Could you check a few things on this model? Use its own coordinates, in mm. Face numbers are marked on the shaded views. A direction names the side the tool comes from. Round coordinates to 2 decimals unless told otherwise and drop trailing zeros. Loops run counter-clockwise (first coordinate to the right, second up) from the corner with the lowest first, then second, coordinate; pieces in that order, holes last. Notation, with made-up numbers: (77, -36) -> (89, -36) arc R18 ccw to (89, -21) -> close; hole circle Ø5 at (64, 45.5). An arc over 180 degrees is marked (long way). One line per item, written item: value.
```python
from build123d import *

# Parameters (mm, degrees)
SKETCH2_R              = 1.5
BOSS_EXTRUDE1_DEPTH    = 8
CHAMFER1_SIZE          = 0.375
CUT_SWEEP1_PITCH       = 0.5
CUT_SWEEP1_HEIGHT      = 8.5
CUT_SWEEP1_RADIUS      = 1.5
CUT_SWEEP1_START_ANGLE = -90
CUT_EXTRUDE1_DEPTH     = 1.62
SKETCH8_R              = 1.154700538
CUT_EXTRUDE2_DEPTH     = 11.0000001
CUT_EXTRUDE2_DRAFT     = -45
SKETCH9_R              = 1.5
BOSS_EXTRUDE2_DEPTH    = 8.38
CHAMFER2_SIZE          = 0.5
CHAMFER2_SIZE2         = 0.866025404


with BuildPart() as part:
    # Sketch2 → Boss-Extrude1 (new body)
    with BuildSketch(Plane(origin=(4, 0, 0), x_dir=(0, 0, -1), z_dir=(1, 0, 0))):
        Circle(SKETCH2_R)
    extrude(amount=-BOSS_EXTRUDE1_DEPTH)

    # Chamfer1
    chamfer1_edges = [part.edges().sort_by_distance(p)[0] for p in [
        (4, 0, 1.5),
    ]]
    chamfer(chamfer1_edges, length=CHAMFER1_SIZE)

    # Cut-Sweep1: sweep along a helix
    with BuildLine() as cut_sweep1_path:
        add(Helix(CUT_SWEEP1_PITCH, CUT_SWEEP1_HEIGHT, CUT_SWEEP1_RADIUS, center=(4, 0, 0), direction=(-1, 0, 0), mode=Mode.PRIVATE).rotate(Axis((4, 0, 0), (-1, 0, 0)), CUT_SWEEP1_START_ANGLE))
    # Sketch5 → Cut-Sweep1 (sweep, cut)
    with BuildSketch(Plane.XY):
        Polygon((3.78125, 1.5), (4.21875, 1.5), (4.03125, 1.175240474), (3.96875, 1.175240474), align=None)
    sweep(path=cut_sweep1_path.line, is_frenet=True, mode=Mode.SUBTRACT)

    # Sketch6 → Revolve1 (revolve)
    with BuildSketch(Plane.XY):
        Polygon((-5.75, 2.75), (-6, 2.5), (-6, 0), (-4, 0), (-4, 2.75), align=None)
    revolve(axis=Axis((-4, 0, 0), (-1, 0, 0)))

    # Sketch4 → Cut-Extrude1 (cut)
    with BuildSketch(Plane(origin=(-6, 0, 0), x_dir=(0, 0, -1), z_dir=(1, 0, 0))):
        Polygon((0, 1.154700538), (-1, 0.577350269), (-1, -0.577350269), (0, -1.154700538), (1, -0.577350269), (1, 0.577350269), align=None)
    extrude(amount=CUT_EXTRUDE1_DEPTH, mode=Mode.SUBTRACT)


with BuildPart() as cut_extrude2_tool:
    # Sketch8 → Cut-Extrude2 (with draft: the straight prism first)
    with BuildSketch(Plane.ZY.offset(6)):
        Circle(SKETCH8_R)
    extrude(amount=-CUT_EXTRUDE2_DEPTH)
    # Cut-Extrude2: the draft: its side faces are tilted about the plane it starts from
    cut_extrude2_sides = [cut_extrude2_tool.faces().sort_by_distance(p)[0] for p in [
        (-0.49999995, 0, -1.154700538),
    ]]
    draft(cut_extrude2_sides, Plane.ZY.offset(6), CUT_EXTRUDE2_DRAFT)


with BuildPart() as part_1:
    add(part.part)

    # Cut-Extrude2: cut by cut_extrude2_tool
    add(cut_extrude2_tool.part, mode=Mode.SUBTRACT)

    # Sketch9 → Boss-Extrude2 (add)
    with BuildSketch(Plane(origin=(4, 0, 0), x_dir=(0, 0, -1), z_dir=(1, 0, 0))):
        Circle(SKETCH9_R)
    extrude(amount=-BOSS_EXTRUDE2_DEPTH)

    # Chamfer2
    chamfer2_edges = [part_1.edges().sort_by_distance(p)[0] for p in [
        (4, 0, 1.5),
    ]]
    chamfer2_side = [part_1.faces().sort_by_distance(p)[0] for p in [
        (0, 0, 1.5),
    ]]
    chamfer(chamfer2_edges, length=CHAMFER2_SIZE, length2=CHAMFER2_SIZE2, reference=chamfer2_side[0])


solid = part_1.part
```
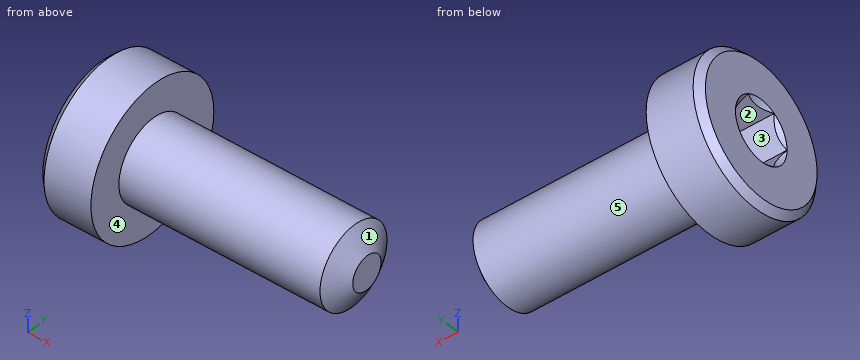
(1) We'd pull the mould along Y, two halves only. Please class the marked faces 3, 4 and 5: +Y half, -Y half, draft (parallel to the pull), parting line (faces both ways), or undercut.
Results below:
face 3: undercut
face 4: draft
face 5: parting line
(2) Imagine slicing it at A-A on y = 0. Write out the boundary of the cut face in (x, z), then the cut area to 3 significant figures.
Results below:
outline: (-6, -2.5) -> (-5.75, -2.75) -> (-4, -2.75) -> (-4, -1.5) -> (3.5, -1.5) -> (4, -0.63) -> (4, 0.63) -> (3.5, 1.5) -> (-4, 1.5) -> (-4, 2.75) -> (-5.75, 2.75) -> (-6, 2.5) -> (-6, 1.15) -> (-5.85, 1) -> (-4.38, 1) -> (-4.38, -1) -> (-5.85, -1) -> (-6, -1.15) -> close
area: 31.2 mm²
(3) Please list where these lines run through material, in increasing order: L1, parallel to X at y = -0.15, z = -1.9; L2, parallel to Z at x = -5.5, y = -0.55; L3, parallel to X at y = 0.15, z = 0.2.
Results below:
L1: x = -6 to -4
L2: z = -2.69 to -1, 1 to 2.69
L3: x = -4.38 to 4
(4) On a 3-axis mill with a long thin cutter (end or side, diameter ignored), from which of +Z, -Z, +X, -X, +Y, -Y can I reach the whole of each face in a straight line? I mean the marked faces 1 and 2. Say none if no direction works.
Results below:
face 1: +X
face 2: -X
(5) Imagine slicing it at B-B on x = -0.25. Write out the boundary of the cut face in (y, z), then the cut area to 3 significant figures.
Results below:
outline: circle Ø3 at (0, 0)
area: 7.07 mm²
(6) For pin 1 Ø1.5 at (x, z) = (0.5, -0.5) entering from +Y; pin 2 Ø1.6 at (y, z) = (-0.5, 0) entering from -X, each with a flat end and sliding along its axis, tell me the tip position at first contact or that it passes through.
Results below:
pin 1: stops at y = 1.5
pin 2: stops at x = -6
